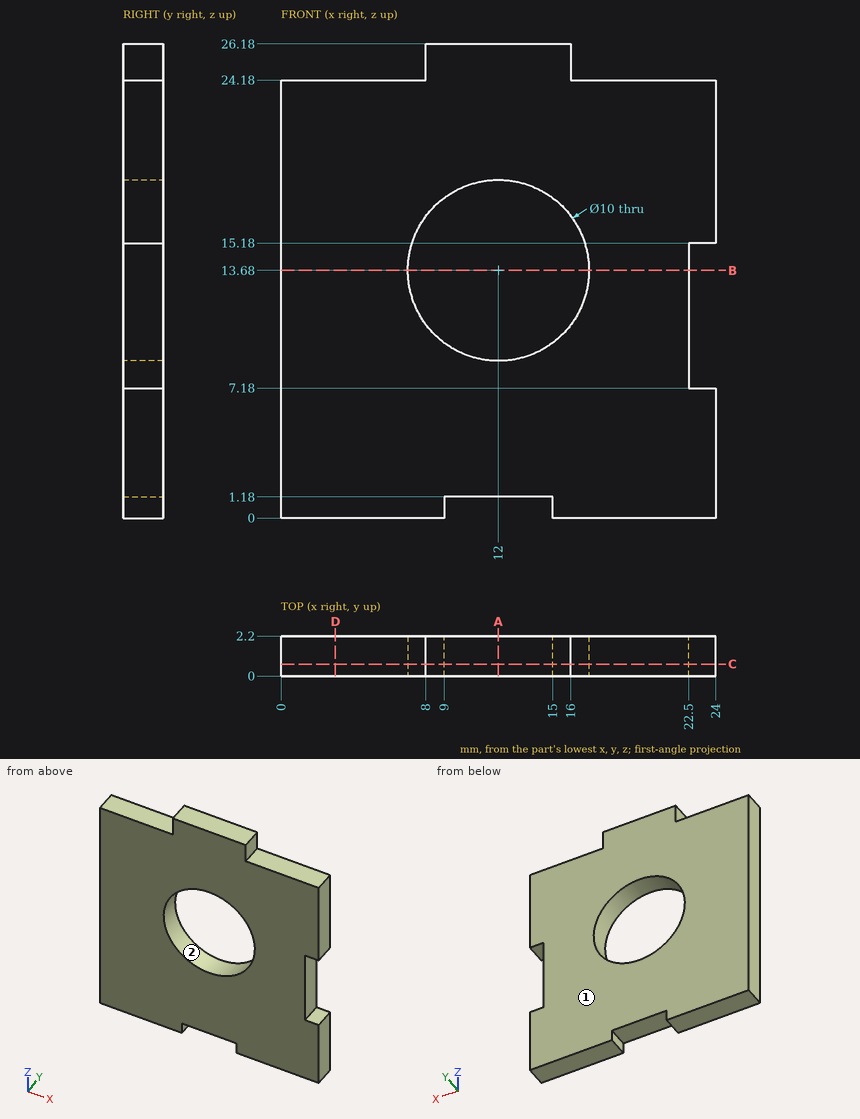
Check sheet for the drawn part. Datum: minimum x, y, z corner. Units: mm. Give positions to 0.01 mm unless a question says otherwise; leave off trailing zeros. Order: outer loops, then holes, each group sorted by start corner. A loop starts at its lowest first (then second) coordinate and runs counter-clockwise, first axis right, second up. Notation, with made-up numbers: (62.5, -23.75) -> (111.5, -23.75) arc R18 cw to (111.5, 3.25) -> close; hole circle Ø6 at (22.25, 14). An arc over 180 degrees is marked (long way). Use a Markdown table: item, result.
1) Section check D-D, the plane x = 3. Record the boundary of the cut face in (y, z).
Results:
| item | result |
|---|---|
| outline | (0, 0) -> (2.2, 0) -> (2.2, 24.18) -> (0, 24.18) -> close |
2) Depth check by flat-ended pin: pin 1 Ø0.7 at (x, y) = (11.5, 1) entering from -Z; pin 2 Ø0.6 at (y, z) = (1, 25) entering from +X. Enter the tip coordinate at first touch or a pass-through.
Results:
| item | result |
|---|---|
| pin 1 | z = 1.18 |
| pin 2 | x = 16 |
3) Section check C-C, the plane y = 0.65. Record the boundary of the cut face in (x, z).
Results:
| item | result |
|---|---|
| outline | (0, 0) -> (9, 0) -> (9, 1.18) -> (15, 1.18) -> (15, 0) -> (24, 0) -> (24, 7.18) -> (22.5, 7.18) -> (22.5, 15.18) -> (24, 15.18) -> (24, 24.18) -> (16, 24.18) -> (16, 26.18) -> (8, 26.18) -> (8, 24.18) -> (0, 24.18) -> close; hole circle Ø10 at (12, 13.68) |
4) Material ranges on probe 1 along X at (y, z) = (0.8, 13.68); probe 2 along Z at (x, y) = (18.75, 1.9); probe 3 along Z at (x, y) = (11.25, 0.8), recorded low to high.
Results:
| item | result |
|---|---|
| probe 1 | 0 to 7, 17 to 22.5 |
| probe 2 | 0 to 24.18 |
| probe 3 | 1.18 to 8.74, 18.62 to 26.18 |
5) Mould release check, pull along X, two halves, no side actions. Record for the marked faces 1 and 2: pulls with the +X half, pulls with the -X half, needs draft (parallel to the pull), parting line crosses it, or undercut.
Results:
| item | result |
|---|---|
| face 1 | needs draft |
| face 2 | undercut |
6) Section check B-B, the plane z = 13.68. Record the boundary of the cut face in (x, y).
Results:
| item | result |
|---|---|
| outline | (0, 0) -> (7, 0) -> (7, 2.2) -> (0, 2.2) -> close; (17, 0) -> (22.5, 0) -> (22.5, 2.2) -> (17, 2.2) -> close |
7) Section check A-A, the plane x = 12. Record the boundary of the cut face in (y, z), then the cut area to 3 significant figures.
Results:
| item | result |
|---|---|
| outline | (0, 1.18) -> (2.2, 1.18) -> (2.2, 8.68) -> (0, 8.68) -> close; (0, 18.68) -> (2.2, 18.68) -> (2.2, 26.18) -> (0, 26.18) -> close |
| area | 33.0 mm² |
